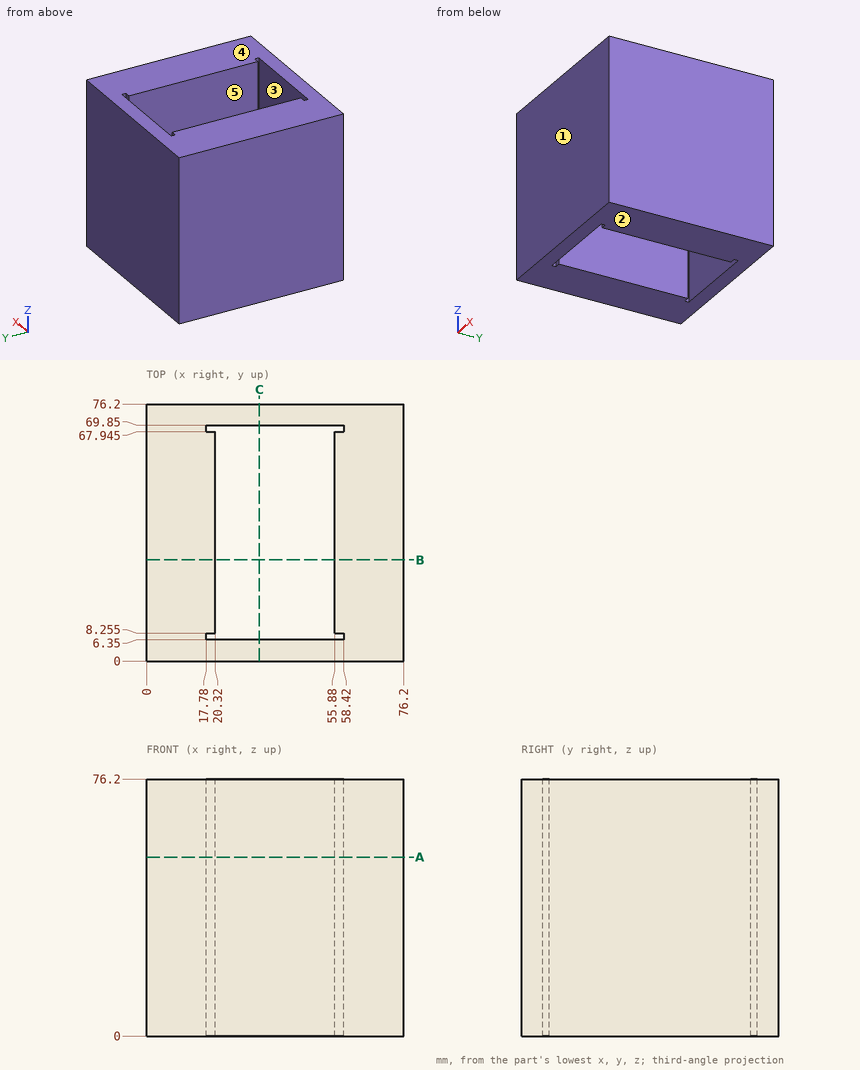
Verification items for this drawing (mm, ordinates from the low corner). A direction names the side the tool comes from. Give positions to 0.01 mm unless a question says otherwise; leave off trailing zeros. Loops run counter-clockwise (first coordinate to the right, second up) from the corner with the lowest first, then second, coordinate; pieces in that order, holes last. Notation, with made-up numbers: M 7.25,-16 L 27.25,-16 A12 ccw 27.25,-11 Z; hole C 25,49 d1. An arc over 180 degrees is marked long. Answer as a JSON object with one key per item and string values. Group by question number.
Item 1: Sectioned sample at A-A on z = 53. Record the boundary of the cut face in (x, y) (3 decimals), plus the area to 3 significant figures.
Item 2: Access from +Z, -Z, +X, -X, +Y, -Y to the whole of each face (thin tool, end or side, straight path). Record for the marked faces 4 and 5.
Item 3: Sectioned sample at C-C on x = 33.5. Record the boundary of the cut face in (y, z), plus the area to 3 significant figures.
Item 4: Sectioned sample at B-B on y = 30. Record the boundary of the cut face in (x, z).
Item 5: Material ranges on L1, parallel to Y at x = 58, z = 4.5 (3 decimals); L2, parallel to X at y = 45.5, z = 8.5; L3, parallel to Y at x = 34, z = 38.5, recorded low to high.
Item 6: Mould release check, pull along Y, two halves, no side actions. Record for the marked faces 1, 2 and 3: pulls with the +Y half, pulls with the -Y half, needs draft (parallel to the pull), parting line crosses it, or undercut.
Findings below:
{
 "1": {"outline": "M 0,0 L 76.2,0 L 76.2,76.2 L 0,76.2 Z; hole M 17.78,6.35 L 58.42,6.35 L 58.42,8.255 L 55.88,8.255 L 55.88,67.945 L 58.42,67.945 L 58.42,69.85 L 17.78,69.85 L 17.78,67.945 L 20.32,67.945 L 20.32,8.255 L 17.78,8.255 Z", "area": "3,530 mm2"},
 "2": {"face 4": "+Z, +X, -X, +Y, -Y", "face 5": "+Z, -Z"},
 "3": {"outline": "M 0,0 L 6.35,0 L 6.35,76.2 L 0,76.2 Z; M 69.85,0 L 76.2,0 L 76.2,76.2 L 69.85,76.2 Z", "area": "968 mm2"},
 "4": {"outline": "M 0,0 L 20.32,0 L 20.32,76.2 L 0,76.2 Z; M 55.88,0 L 76.2,0 L 76.2,76.2 L 55.88,76.2 Z"},
 "5": {"L1": "0 to 6.35, 8.255 to 67.945, 69.85 to 76.2", "L2": "0 to 20.32, 55.88 to 76.2", "L3": "0 to 6.35, 69.85 to 76.2"},
 "6": {"face 1": "pulls with the -Y half", "face 2": "needs draft", "face 3": "undercut"}
}
